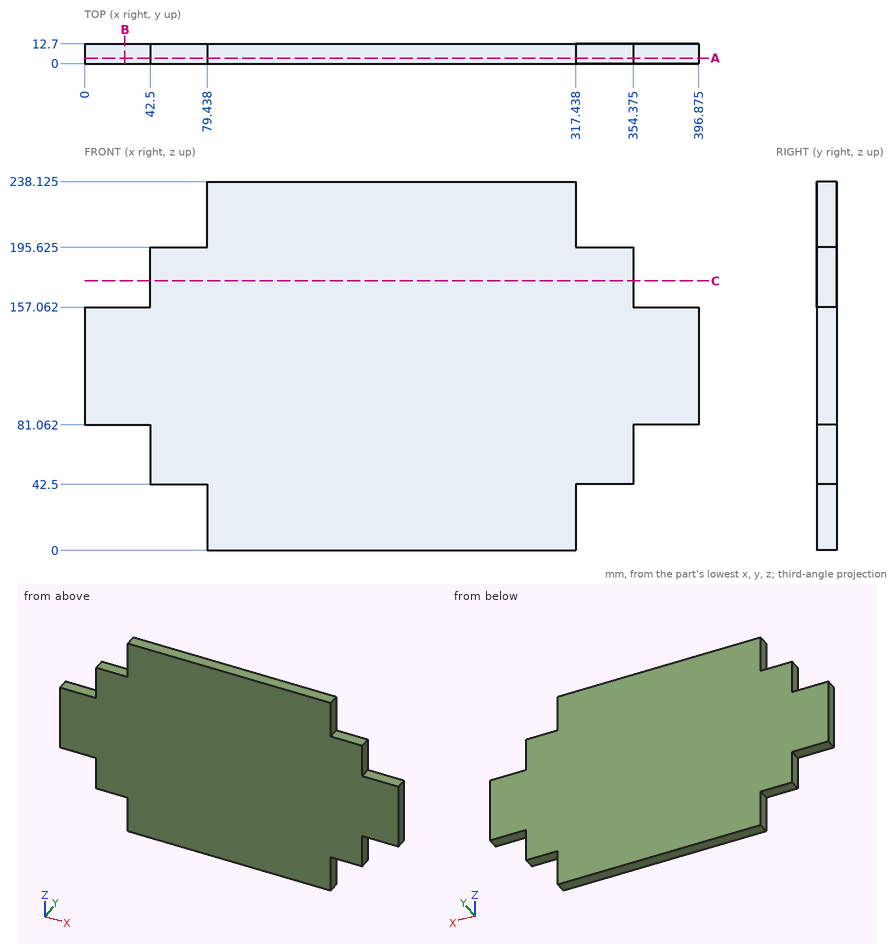
Job drawing, mm, ordinate dimensions from the low corner. One solid piece. Give positions to 0.01 mm unless a question says otherwise; leave off trailing zeros. Write each loop counter-clockwise with the first axis right and the second up, starting at its lowest first coordinate (ties: lowest second). Pieces come first, ordered by that corner, then holes. Notation, with made-up numbers: (39.25, 84.25) - (52.25, 84.25) arc R33 cw to (52.25, 120.25) - close; hole circle Ø3 at (25.5, 79). An arc over 180 degrees is marked (long way). Answer as CSV lines item,"result".
1. Band-saw the part on C-C (z = 174). Write the cut outline in (x, y) (1 decimal), and give its area (3 significant figures).
Responses:
outline,"(42.5, 0) - (354.4, 0) - (354.4, 12.7) - (42.5, 12.7) - close"
area,"3,960 mm2"
2. Drill centre lines: L1, parallel to X at y = 10, z = 38.5; L2, parallel to X at y = 2, z = 65.5 (1 decimal); L3, parallel to Z at x = 49.5, y = 7.25 (1 decimal). Where is each one in solid material? Low to high. Write a range as [from, to].
Responses:
L1,"x = [79.44, 317.44]"
L2,"x = [42.5, 354.4]"
L3,"z = [42.5, 195.6]"
3. Band-saw the part on A-A (y = 3.5). Write the cut outline in (x, z) (1 decimal).
Responses:
outline,"(0, 81.1) - (42.5, 81.1) - (42.5, 42.5) - (79.4, 42.5) - (79.4, 0) - (317.4, 0) - (317.4, 42.5) - (354.4, 42.5) - (354.4, 81.1) - (396.9, 81.1) - (396.9, 157.1) - (354.4, 157.1) - (354.4, 195.6) - (317.4, 195.6) - (317.4, 238.1) - (79.4, 238.1) - (79.4, 195.6) - (42.5, 195.6) - (42.5, 157.1) - (0, 157.1) - close"
4. Band-saw the part on B-B (x = 26). Write the cut outline in (y, z).
Responses:
outline,"(0, 81.06) - (12.7, 81.06) - (12.7, 157.06) - (0, 157.06) - close"
5. Pin check, flat tips, straight feed: pin 1 (6.5 mm diameter, centred on y = 8.5, z = 178.5, fed in from +X) (1 decimal); pin 2 (6.5 mm diameter, centred on x = 59, y = 8, fed in from -Z); pin 3 (6.5 mm diameter, centred on y = 8, z = 217.5, fed in from +X); pin 4 (1 mm diameter, centred on x = 203.5, y = 4.5, fed in from -Z). Stop position of each tip, or through.
Responses:
pin 1,"stops at x = 354.4"
pin 2,"stops at z = 42.5"
pin 3,"stops at x = 317.44"
pin 4,"stops at z = 0"
